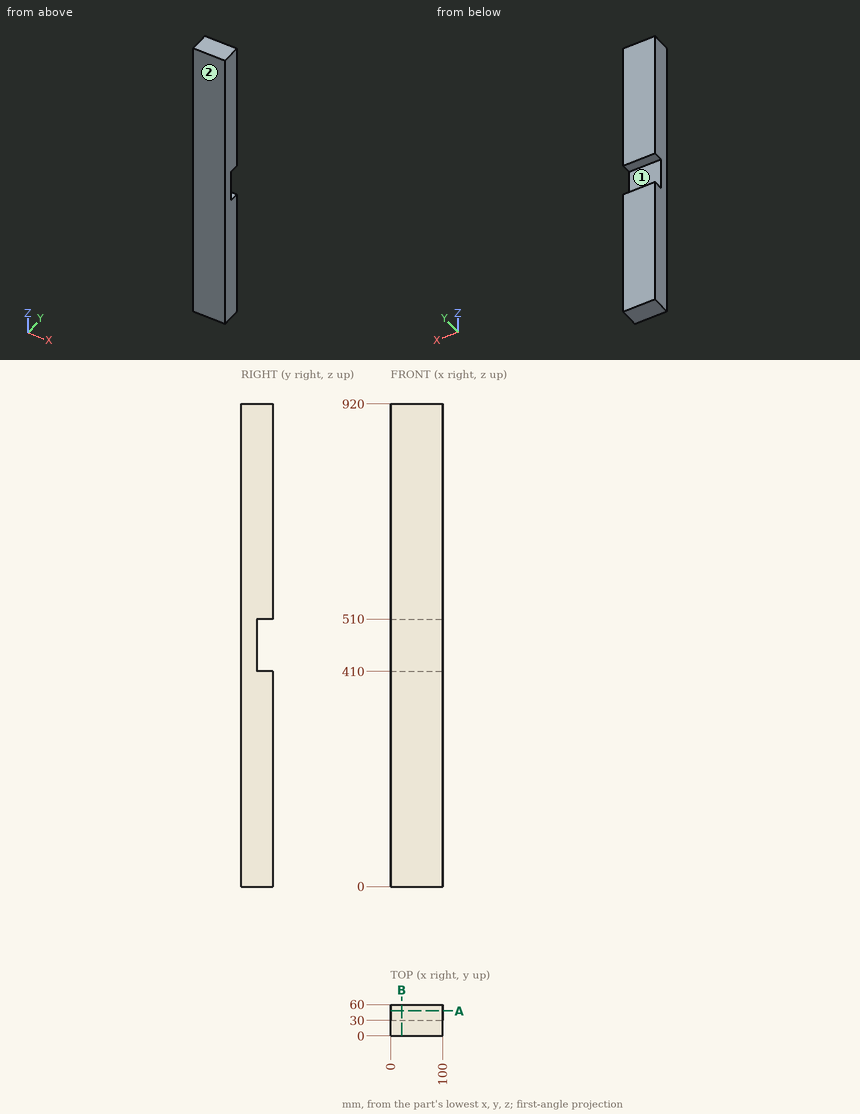
Verification items for this drawing (mm, ordinates from the low corner). Coordinates: 2 decimals unless noted, no trailing zeros. Write each loop counter-clockwise with the first axis right and the second up, starting at its lowest first coordinate (ties: lowest second). Pieces come first, ordered by that corner, then holes. Notation, with made-up numbers: M 37,22 L 57,22 A34 ccw 57,54 Z; hole C 43.5,-25.5 d10. An arc over 180 degrees is marked long. Answer as a JSON object with one key per item and string values.
1. Scan lines: L1, parallel to Z at x = 80, y = 54; L2, parallel to Y at x = 96.5, z = 460. Record each from-to range of solid material in increasing order.
Answers below:
{"L1": "z = 0 to 410, 510 to 920", "L2": "y = 0 to 30"}
2. Section check A-A, the plane y = 48. Enter the section's corners in (x, z).
Answers below:
{"outline": "M 0,0 L 100,0 L 100,410 L 0,410 Z; M 0,510 L 100,510 L 100,920 L 0,920 Z"}
3. Draft check along Z on the marked faces 1 and 2. Enter one of: released by +Z, released by -Z, zero draft, split by the parting line, or undercut.
Answers below:
{"face 1": "undercut", "face 2": "zero draft"}
4. Section check B-B, the plane x = 21. Enter the section's corners in (y, z).
Answers below:
{"outline": "M 0,0 L 60,0 L 60,410 L 30,410 L 30,510 L 60,510 L 60,920 L 0,920 Z"}
